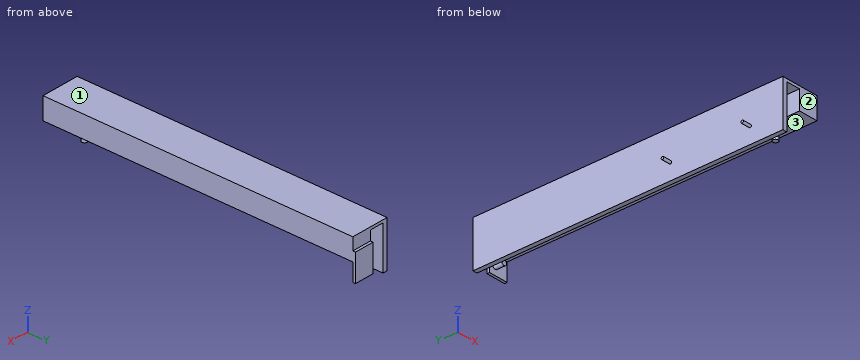
```python
from build123d import *

# Parameters (mm, degrees)
F0_W      = 3
F0_H      = 350
F1_DEPTH  = 52
F2_W      = 350
F2_H      = 3
F3_DEPTH  = 40
F4_W      = 22
F4_H      = 350
F5_DEPTH  = 21.5
F6_R      = 1.5
F7_DEPTH  = 10
F8_W      = 22
F8_H      = 10.75
F9_DEPTH  = 3
F10_DEPTH = 20
F11_R     = 3
F12_DEPTH = 10
F13_R     = 3
F14_DEPTH = 10
F15_DEPTH = 2


with BuildPart() as f1:
    # F0 (on Top) → F1 (new body)
    with BuildSketch(Plane.XY):
        with Locations((-1.5, 0)):
            Rectangle(F0_W, F0_H)
    extrude(amount=F1_DEPTH)

    # F2 (on face) → F3 (join)
    with BuildSketch(Plane.YZ):
        with Locations((0, 50.5)):
            Rectangle(F2_W, F2_H)
    extrude(amount=F3_DEPTH)

    # F4 (on face) → F5 (join)
    with BuildSketch(Plane(origin=(0, 0, 49), x_dir=(1, 0, 0), z_dir=(0, 0, -1))):
        with Locations((29, 0)):
            Rectangle(F4_W, F4_H)
    extrude(amount=F5_DEPTH)

    # F6 (on face) → F7 (join)
    with BuildSketch(Plane(origin=(-3, 0, 0), x_dir=(0, -1, 0), z_dir=(-1, 0, 0))):
        with Locations((138, 18)):
            Circle(F6_R)
        with Locations((48, 18)):
            Circle(F6_R)
    extrude(amount=F7_DEPTH)



with BuildPart() as f9:
    # F8 (on face) → F9 (new body)
    with BuildSketch(Plane(origin=(0, 175, 0), x_dir=(-1, 0, 0), z_dir=(0, 1, 0))):
        with Locations((-29, 32.875)):
            Rectangle(F8_W, F8_H)
    extrude(amount=F9_DEPTH)


with BuildPart() as f1_1:
    add(f1.part)
    # F10 (add): a face of the model
    f10_faces = [f9.part.faces().sort_by_distance(p)[0] for p in [
        (29, 176.5, 27.5),
    ]]

    add(f9.part)  # F10 merges F9
    extrude(f10_faces, amount=F10_DEPTH)

    # F11 (on face) → F12 (join)
    with BuildSketch(Plane.XZ.offset(-175)):
        with Locations((25, 16.5)):
            Circle(F11_R)
    extrude(amount=F12_DEPTH)

    # F13 (on face) → F14 (join)
    with BuildSketch(Plane(origin=(0, 0, 27.5), x_dir=(1, 0, 0), z_dir=(0, 0, -1))):
        with Locations((29, 138)):
            Circle(F13_R)
    extrude(amount=F14_DEPTH)

    # F15 (add): a face of the model
    f15_faces = [f1_1.faces().sort_by_distance(p)[0] for p in [
        (0, 0, 24.5),
    ]]
    extrude(f15_faces, amount=F15_DEPTH)


solid = f1_1.part
```
The listing builds one solid part. Answer for the finished solid, in the listing's coordinates (mm). Face numbers are marked on the shaded views. Give positions to 0.01 mm unless a question says otherwise; leave off trailing zeros. Order: outer loops, then holes, each group sorted by start corner. A loop starts at its lowest first (then second) coordinate and runs counter-clockwise, first axis right, second up. Notation, with made-up numbers: (30, 12) - (44, 12) arc R22 cw to (44, 24) - close; hole circle Ø1 at (39, -16). An arc over 180 degrees is marked (long way). Use one line per item in the form item = value. Start each with the question number.
(1) A cutting plane is placed at C-C, the plane y = -12. Write down the section's boundary in (x, z).
(2) A cutting plane is placed at D-D, the plane z = 4. Write down the section's boundary in (x, y), then the cut area to 3 significant figures.
(3) The mould has two halves that part along Y. Classify the marked faces 1, 2 and 3: released by +Y, released by -Y, zero draft, split by the parting line, or undercut.
(4) A cutting plane is placed at A-A, the plane z = 41.5. Write down the section's boundary in (x, y).
(5) A cutting plane is placed at B-B, the plane x = 35. Write down the section's boundary in (y, z), then the cut area to 3 significant figures.
(6) Consider line 1 (X direction, y = 162, z = 30); line 2 (X direction, y = -154.5, z = 6); line 3 (Z direction, x = 15, y = 92.5). Determine where each line is inside the solid, lowest interval first. Write a range as from..to.
(7) Flat-ended cylindrical pins translate along their axes: pin 1 Ø15.5 at (y, z) = (86, 24) entering from -X; pin 2 Ø13 at (x, y) = (10.5, 42) entering from -Z; pin 3 Ø0.9 at (x, y) = (26.5, 177) entering from -Z; pin 4 Ø12 at (x, z) = (12.5, 19) entering from +Y. Find the tip coordinate at first contact, or state that the pin passes through.
Ans:
q1.outline = (-3, 0) - (2, 0) - (2, 49) - (18, 49) - (18, 27.5) - (40, 27.5) - (40, 52) - (-3, 52) - close
q2.outline = (-3, -175) - (2, -175) - (2, 175) - (-3, 175) - close
q2.area = 1,750 mm^2
q3.face_1 = zero draft
q3.face_2 = released by -Y
q3.face_3 = undercut
q4.outline = (-3, -175) - (2, -175) - (2, 175) - (-3, 175) - close; (18, -175) - (40, -175) - (40, 175) - (18, 175) - close
q5.outline = (-175, 27.5) - (175, 27.5) - (175, 7.5) - (178, 7.5) - (178, 38.25) - (175, 38.25) - (175, 52) - (-175, 52) - close
q5.area = 8,670 mm^2
q6.line_1 = -3..2, 18..40
q6.line_2 = -3..2
q6.line_3 = 49..52
q7.pin_1 = -3
q7.pin_2 = 49
q7.pin_3 = 7.5
q7.pin_4 = 178
